The listing builds one solid part. Answer for the finished solid, in the listing's coordinates (mm). Give positions to 0.01 mm unless a question says otherwise; leave off trailing zeros. Loops run counter-clockwise (first coordinate to the right, second up) from the corner with the lowest first, then second, coordinate; pieces in that order, holes last.
Item 1: Section C-C, the plane y = 1.6 is taken. Give the vertices of the cut face in (x, z), and give its area (3 significant figures).
Item 2: Consider line 1 along X through (y, z) = (1.7, -12.5); line 2 along Z through (x, y) = (89, 2.7); line 3 along Z through (x, y) = (20, 1.9). Determine where each line is inside the solid, lowest interval first.
Item 3: Section D-D, the plane z = -2.75 is taken. Give the vertices of the cut face in (x, y).
Item 4: Section A-A, the plane x = 20 is taken. Give the vertices of the cut face in (y, z), and give its area (3 significant figures).
Item 5: Section B-B, the plane z = -9.25 is taken. Give the vertices of the cut face in (x, y).
Item 6: Each of these flat-tipped pins is pushed along its axis until it touches: pin 1 Ø1.5 at (y, z) = (1, -4) entering from +X; pin 2 Ø0.9 at (y, z) = (1.5, -14) entering from +X. Where does it stop, or does it pass through?
from build123d import *

# Parameters (mm, degrees)
SKETCH1_W           = 110
SKETCH1_H           = 25
BOSS_EXTRUDE1_DEPTH = 3
SKETCH2_W           = 23
SKETCH2_H           = 12
CUT_EXTRUDE1_DEPTH  = 4
SKETCH3_R           = 1
CUT_EXTRUDE2_DEPTH  = 4
FILLET1_R           = 12


with BuildPart() as part:
    # Sketch1 → Boss-Extrude1 (new body)
    with BuildSketch(Plane(origin=(0, 0, 0), x_dir=(1, 0, 0), z_dir=(0, 1, 0))):
        with Locations((55, 12.5)):
            Rectangle(SKETCH1_W, SKETCH1_H)
    extrude(amount=BOSS_EXTRUDE1_DEPTH)

    # Sketch2 → Cut-Extrude1 (cut, through all)
    with BuildSketch(Plane(origin=(0, 3, 0), x_dir=(1, 0, 0), z_dir=(0, 1, 0))):
        with Locations((84.5, 12.5)):
            Rectangle(SKETCH2_W, SKETCH2_H)
    extrude(amount=-CUT_EXTRUDE1_DEPTH, mode=Mode.SUBTRACT)

    # Sketch3 → Cut-Extrude2 (cut, through all)
    with BuildSketch(Plane(origin=(0, 3, 0), x_dir=(1, 0, 0), z_dir=(0, 1, 0))):
        with Locations((20, 12.5)):
            Circle(SKETCH3_R)
    extrude(amount=-CUT_EXTRUDE2_DEPTH, mode=Mode.SUBTRACT)

    # Fillet1
    fillet1_edges = [part.edges().sort_by_distance(p)[0] for p in [
        (0, 1.5, -25),
        (110, 1.5, -25),
        (110, 1.5, 0),
        (0, 1.5, 0),
    ]]
    fillet(fillet1_edges, radius=FILLET1_R)


solid = part.part
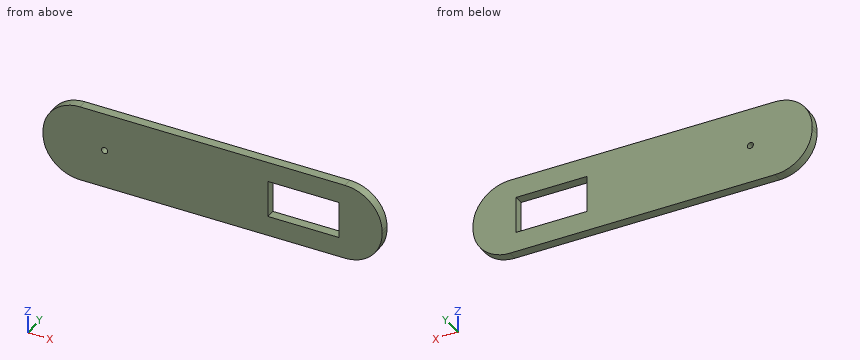
Worked answers:
1. outline: (0, -13) arc R12 ccw to (12, -25) - (98, -25) arc R12 ccw to (110, -13) - (110, -12) arc R12 ccw to (98, 0) - (12, 0) arc R12 ccw to (0, -12) - close; hole circle Ø2 at (20, -12.5); hole (73, -18.5) - (96, -18.5) - (96, -6.5) - (73, -6.5) - close
1. area: 2,350 mm2
2. line 1: x = 0 to 19, 21 to 73, 96 to 110
2. line 2: z = -25 to -18.5, -6.5 to 0
2. line 3: z = -25 to -13.5, -11.5 to 0
3. outline: (4.36, 0) - (105.64, 0) - (105.64, 3) - (4.36, 3) - close
4. outline: (0, -25) - (3, -25) - (3, -13.5) - (0, -13.5) - close; (0, -11.5) - (3, -11.5) - (3, 0) - (0, 0) - close
4. area: 69.0 mm2
5. outline: (0.32, 0) - (73, 0) - (73, 3) - (0.32, 3) - close; (96, 0) - (109.68, 0) - (109.68, 3) - (96, 3) - close
6. pin 1: stops at x = 107.56
6. pin 2: stops at x = 109.99
